Work out the finished part from the listing and answer in its coordinate system (mm). A direction names the side the tool comes from. Round coordinates to 2 decimals unless told otherwise and drop trailing zeros. Write each loop counter-clockwise with the first axis right and the second up, starting at its lowest first coordinate (ties: lowest second). Pieces come first, ordered by that corner, then holes. Notation, with made-up numbers: M 9.25,-23 L 48.25,-23 A35 ccw 48.25,11 Z; hole C 86,57.5 d5. An arc over 180 degrees is marked long. One line per item, written item: value. Start each with the question number.
Q1. The mould has two halves that part along Y. Classify faces 1 (the cylindrical face through (13.5, 0, 3)), 2 (the cylindrical face through (7.48, 12.27, 2.99)), 3 (the flat face through (0, 0, 0)): released by +Y, released by -Y, zero draft, split by the parting line, or undercut.
Q2. Find section A-A (x = 0). Write down the section's boundary in (y, z).
Q3. Consider probe 1 along Y at (x, z) = (0, 3.65); probe 2 along Y at (x, z) = (-0.25, 0.8); probe 3 along Z at (x, y) = (-6, 0.5). Determine where each line is inside the solid, lowest interval first.
Q4. Given pin 1 Ø6 at (x, y) = (5, -1) entering from +Z; pin 2 Ø2 at (y, z) = (-5, 1) entering from +X; pin 3 Ø1.5 at (x, z) = (8, 3) entering from +Y, each flat-ended and moving along its own axis, determine where each tip first touches the part or whether it passes through.
Q5. Find section B-B (y = -7). Write down the section's boundary in (x, z).
Q6. Find section C-C (z = 1.3). Write down the section's boundary in (x, y).
Q7. Find section D-D (y = -14). Write down the section's boundary in (x, z).
Q8. A tool of negligible diameter and unlimited length cuts with its end or side. For faces 4 (the flat face through (0, -14, 4)), 5 (the cylindrical face through (12.02, 6.51, 2.99)), from which of +Z, -Z, +X, -X, +Y, -Y can it reach the whole face along a straight path? Write none if from no direction.
from build123d import *

# Parameters (mm, degrees)
F0_R     = 15
F1_DEPTH = 2
F2_R     = 0.5
F3_DEPTH = 2


with BuildPart() as f1:
    # F0 (on Top) → F1 (new body)
    with BuildSketch(Plane.XY):
        Circle(F0_R)
    extrude(amount=F1_DEPTH)

    # F2 (on face) → F3 (join)
    with BuildSketch(Plane.XY.offset(2)):
        with Locations((0, 14)):
            Circle(F2_R)
        with Locations((7, 12.124356)):
            Circle(F2_R)
        with Locations((12.124356, 7)):
            Circle(F2_R)
        with Locations((14, 0)):
            Circle(F2_R)
        with Locations((12.124356, -7)):
            Circle(F2_R)
        with Locations((7, -12.124356)):
            Circle(F2_R)
        with Locations((0, -14)):
            Circle(F2_R)
        with Locations((-7, -12.124356)):
            Circle(F2_R)
        with Locations((-12.124356, -7)):
            Circle(F2_R)
        with Locations((-14, 0)):
            Circle(F2_R)
        with Locations((-12.124356, 7)):
            Circle(F2_R)
        with Locations((-7, 12.124356)):
            Circle(F2_R)
    extrude(amount=F3_DEPTH)


solid = f1.part
The answers:
1. face 1: split by the parting line
1. face 2: undercut
1. face 3: zero draft
2. outline: M -15,0 L 15,0 L 15,2 L 14.5,2 L 14.5,4 L 13.5,4 L 13.5,2 L -13.5,2 L -13.5,4 L -14.5,4 L -14.5,2 L -15,2 Z
3. probe 1: -14.5 to -13.5, 13.5 to 14.5
3. probe 2: -15 to 15
3. probe 3: 0 to 2
4. pin 1: z = 2
4. pin 2: x = 14.46
4. pin 3: y = 12.56
5. outline: M -13.27,0 L 13.27,0 L 13.27,2 L 12.62,2 L 12.62,4 L 11.62,4 L 11.62,2 L -11.62,2 L -11.62,4 L -12.62,4 L -12.62,2 L -13.27,2 Z
6. outline: C 0,0 d30
7. outline: M -5.39,0 L 5.39,0 L 5.39,2 L 0.5,2 L 0.5,4 L -0.5,4 L -0.5,2 L -5.39,2 Z
8. face 4: +Z, +X, -X, +Y, -Y
8. face 5: +Z
